Read the model definition and answer for the solid it produces. Units are mm, in the model's axes. A direction names the side the tool comes from. Give positions to 0.01 mm unless a question says otherwise; leave off trailing zeros. Loops run counter-clockwise (first coordinate to the right, second up) from the corner with the lowest first, then second, coordinate; pieces in that order, holes last. Notation, with made-up numbers: (-8.5, 83) -> (24.5, 83) arc R15 cw to (24.5, 96) -> close; hole circle Ø8 at (-16.75, 41). An arc over 180 degrees is marked (long way). Answer as CSV lines item,"result". Start each with the question number.
```python
from build123d import *

# Parameters (mm, degrees)
F1_DEPTH = 5


with BuildPart() as f1:
    # F0 (on Top) → F1 (new body)
    with BuildSketch(Plane.XY):
        with BuildLine():
            Line((-0.474925, 13.057005), (-1.233272, 10.753499))
            ThreePointArc((-1.233272, 10.753499), (-1.642562, 10.370728), (-2.150102, 10.608287))
            Line((-2.150102, 10.608287), (-3.583156, 12.564709))
            ThreePointArc((-3.583156, 12.564709), (-4.141029, 12.744778), (-4.486517, 12.271189))
            Line((-4.486517, 12.271189), (-4.495926, 9.846083))
            ThreePointArc((-4.495926, 9.846083), (-4.7669, 9.355569), (-5.32301, 9.424663))
            Line((-5.32301, 9.424663), (-7.290492, 10.842493))
            ThreePointArc((-7.290492, 10.842493), (-7.876706, 10.841355), (-8.058937, 10.284185))
            Line((-8.058937, 10.284185), (-7.318486, 7.974864))
            ThreePointArc((-7.318486, 7.974864), (-7.424621, 7.424621), (-7.974864, 7.318486))
            Line((-7.974864, 7.318486), (-10.284185, 8.058937))
            ThreePointArc((-10.284185, 8.058937), (-10.841355, 7.876706), (-10.842493, 7.290492))
            Line((-10.842493, 7.290492), (-9.424663, 5.32301))
            ThreePointArc((-9.424663, 5.32301), (-9.355569, 4.7669), (-9.846083, 4.495926))
            Line((-9.846083, 4.495926), (-12.271189, 4.486517))
            ThreePointArc((-12.271189, 4.486517), (-12.744778, 4.141029), (-12.564709, 3.583156))
            Line((-12.564709, 3.583156), (-10.608287, 2.150102))
            ThreePointArc((-10.608287, 2.150102), (-10.370728, 1.642562), (-10.753499, 1.233272))
            Line((-10.753499, 1.233272), (-13.057005, 0.474925))
            ThreePointArc((-13.057005, 0.474925), (-13.400652, 0), (-13.057005, -0.474925))
            Line((-13.057005, -0.474925), (-10.753499, -1.233272))
            ThreePointArc((-10.753499, -1.233272), (-10.370728, -1.642562), (-10.608287, -2.150102))
            Line((-10.608287, -2.150102), (-12.564709, -3.583156))
            ThreePointArc((-12.564709, -3.583156), (-12.744778, -4.141029), (-12.271189, -4.486517))
            Line((-12.271189, -4.486517), (-9.846083, -4.495926))
            ThreePointArc((-9.846083, -4.495926), (-9.355569, -4.7669), (-9.424663, -5.32301))
            Line((-9.424663, -5.32301), (-10.842493, -7.290492))
            ThreePointArc((-10.842493, -7.290492), (-10.841355, -7.876706), (-10.284185, -8.058937))
            Line((-10.284185, -8.058937), (-7.974864, -7.318486))
            ThreePointArc((-7.974864, -7.318486), (-7.424621, -7.424621), (-7.318486, -7.974864))
            Line((-7.318486, -7.974864), (-8.058937, -10.284185))
            ThreePointArc((-8.058937, -10.284185), (-7.876706, -10.841355), (-7.290492, -10.842493))
            Line((-7.290492, -10.842493), (-5.32301, -9.424663))
            ThreePointArc((-5.32301, -9.424663), (-4.7669, -9.355569), (-4.495926, -9.846083))
            Line((-4.495926, -9.846083), (-4.486517, -12.271189))
            ThreePointArc((-4.486517, -12.271189), (-4.141029, -12.744778), (-3.583156, -12.564709))
            Line((-3.583156, -12.564709), (-2.150102, -10.608287))
            ThreePointArc((-2.150102, -10.608287), (-1.642562, -10.370728), (-1.233272, -10.753499))
            Line((-1.233272, -10.753499), (-0.474925, -13.057005))
            ThreePointArc((-0.474925, -13.057005), (0, -13.400652), (0.474925, -13.057005))
            Line((0.474925, -13.057005), (1.233272, -10.753499))
            ThreePointArc((1.233272, -10.753499), (1.642562, -10.370728), (2.150102, -10.608287))
            Line((2.150102, -10.608287), (3.583156, -12.564709))
            ThreePointArc((3.583156, -12.564709), (4.141029, -12.744778), (4.486517, -12.271189))
            Line((4.486517, -12.271189), (4.495926, -9.846083))
            ThreePointArc((4.495926, -9.846083), (4.7669, -9.355569), (5.32301, -9.424663))
            Line((5.32301, -9.424663), (7.290492, -10.842493))
            ThreePointArc((7.290492, -10.842493), (7.876706, -10.841355), (8.058937, -10.284185))
            Line((8.058937, -10.284185), (7.318486, -7.974864))
            ThreePointArc((7.318486, -7.974864), (7.424621, -7.424621), (7.974864, -7.318486))
            Line((7.974864, -7.318486), (10.284185, -8.058937))
            ThreePointArc((10.284185, -8.058937), (10.841355, -7.876706), (10.842493, -7.290492))
            Line((10.842493, -7.290492), (9.424663, -5.32301))
            ThreePointArc((9.424663, -5.32301), (9.355569, -4.7669), (9.846083, -4.495926))
            Line((9.846083, -4.495926), (12.271189, -4.486517))
            ThreePointArc((12.271189, -4.486517), (12.744778, -4.141029), (12.564709, -3.583156))
            Line((12.564709, -3.583156), (10.608287, -2.150102))
            ThreePointArc((10.608287, -2.150102), (10.370728, -1.642562), (10.753499, -1.233272))
            Line((10.753499, -1.233272), (13.057005, -0.474925))
            ThreePointArc((13.057005, -0.474925), (13.400652, 0), (13.057005, 0.474925))
            Line((13.057005, 0.474925), (10.753499, 1.233272))
            ThreePointArc((10.753499, 1.233272), (10.370728, 1.642562), (10.608287, 2.150102))
            Line((10.608287, 2.150102), (12.564709, 3.583156))
            ThreePointArc((12.564709, 3.583156), (12.744778, 4.141029), (12.271189, 4.486517))
            Line((12.271189, 4.486517), (9.846083, 4.495926))
            ThreePointArc((9.846083, 4.495926), (9.355569, 4.7669), (9.424663, 5.32301))
            Line((9.424663, 5.32301), (10.842493, 7.290492))
            ThreePointArc((10.842493, 7.290492), (10.841355, 7.876706), (10.284185, 8.058937))
            Line((10.284185, 8.058937), (7.974864, 7.318486))
            ThreePointArc((7.974864, 7.318486), (7.424621, 7.424621), (7.318486, 7.974864))
            Line((7.318486, 7.974864), (8.058937, 10.284185))
            ThreePointArc((8.058937, 10.284185), (7.876706, 10.841355), (7.290492, 10.842493))
            Line((7.290492, 10.842493), (5.32301, 9.424663))
            ThreePointArc((5.32301, 9.424663), (4.7669, 9.355569), (4.495926, 9.846083))
            Line((4.495926, 9.846083), (4.486517, 12.271189))
            ThreePointArc((4.486517, 12.271189), (4.141029, 12.744778), (3.583156, 12.564709))
            Line((3.583156, 12.564709), (2.150102, 10.608287))
            ThreePointArc((2.150102, 10.608287), (1.642562, 10.370728), (1.233272, 10.753499))
            Line((1.233272, 10.753499), (0.474925, 13.057005))
            ThreePointArc((0.474925, 13.057005), (0, 13.400652), (-0.474925, 13.057005))
        make_face()
    extrude(amount=F1_DEPTH)


solid = f1.part
```
(1) Find section B-B on x = -5.75. Write down the section's boundary in (y, z).
(2) This flat-tipped pin is pushed along its axis until it touches: P1, Ø1, axis at y = 10.5, z = 3, coming from the +X side. Where does it stop, or does it pass through?
(3) The mould has two halves that part along Y. Classify faces 5 (the face through (10.372, 1.634, 2.465)), 6 (the face through (0.85, -11.92, 2.46)), 7 (the face through (-4.13, 12.75, 2.46)), 8 (the face through (-11.89, 0.86, 2.46)): pulls with the +Y half, pulls with the -Y half, needs draft (parallel to the pull), parting line crosses it, or undercut.
(4) Find section A-A on y = 1.75. Write down the section's boundary in (x, z).
(5) Find the intervals of material crossed by line 1 along Y through (x, z) = (10.25, 3.4); line 2 along Y through (x, z) = (9.75, 4.7), in increasing order. Write a range as from..to.
(6) A tool of negligible diameter and unlimited length cuts with its end or side. For faces 1 (the face through (11.573, 2.857, 2.465)), 2 (the face through (-6.321, -10.144, 2.465)), 3 (the face through (-11.92, -0.85, 2.46)), 4 (the face through (-2.857, 11.573, 2.465)), from which of +Z, -Z, +X, -X, +Y, -Y can it reach the whole face along a straight path? Write none if from no direction.
Answer block:
1,outline,"(-9.73, 0) -> (9.73, 0) -> (9.73, 5) -> (-9.73, 5) -> close"
2,P1,"stops at x = 8.08"
3,face 5,"undercut"
3,face 6,"pulls with the -Y half"
3,face 7,"pulls with the +Y half"
3,face 8,"undercut"
4,outline,"(-10.37, 0) -> (10.37, 0) -> (10.37, 5) -> (-10.37, 5) -> close"
5,line 1,"y = -8.05..-6.47, -4.49..4.49, 6.47..8.05"
5,line 2,"y = -7.89..-5.77, -4.5..4.5, 5.77..7.89"
6,face 1,"+Z, -Z, +X"
6,face 2,"+Z, -Z, -Y"
6,face 3,"+Z, -Z, -X"
6,face 4,"+Z, -Z, +Y"
